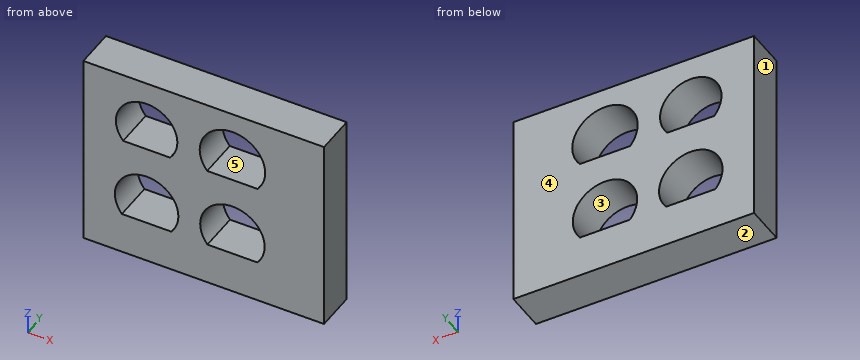
from build123d import *

# Parameters (mm, degrees)
SKETCH1_W           = 12.136372274
SKETCH1_H           = 9.961646607
BOSS_EXTRUDE2_DEPTH = 2


with BuildPart() as part:
    # Sketch1 → Boss-Extrude2 (new body)
    with BuildSketch(Plane(origin=(0, 0, 0), x_dir=(1, 0, 0), z_dir=(0, 1, 0))):
        with Locations((2.877549337, 2.284027555)):
            Rectangle(SKETCH1_W, SKETCH1_H)
        with BuildLine():
            Line((-1.184271928, 1), (1.184271928, 1))
            ThreePointArc((1.184271928, 1), (0, -1.55), (-1.184271928, 1))
        make_face(mode=Mode.SUBTRACT)
        with BuildLine():
            Line((3.05341377, 1), (5.598998182, 1))
            ThreePointArc((5.598998182, 1), (4.326205976, -1.7), (3.05341377, 1))
        make_face(mode=Mode.SUBTRACT)
        with BuildLine():
            Line((-1.2489996, 5.143134086), (1.2489996, 5.143134086))
            ThreePointArc((1.2489996, 5.143134086), (0, 2.543134086), (-1.2489996, 5.143134086))
        make_face(mode=Mode.SUBTRACT)
        with BuildLine():
            Line((3.065253955, 5.143134086), (5.587157997, 5.143134086))
            ThreePointArc((5.587157997, 5.143134086), (4.326205976, 2.493134086), (3.065253955, 5.143134086))
        make_face(mode=Mode.SUBTRACT)
    extrude(amount=BOSS_EXTRUDE2_DEPTH)


solid = part.part
Could you check a few things on this model? Use its own coordinates, in mm. Face numbers are marked on the shaded views. A direction names the side the tool comes from. Give positions to 0.01 mm unless a question says otherwise; leave off trailing zeros. Loops run counter-clockwise (first coordinate to the right, second up) from the corner with the lowest first, then second, coordinate; pieces in that order, holes last. Notation, with made-up numbers: M 7.5,-3 L 40.5,-3 A25 ccw 40.5,9 Z; hole C -24,43 d11. An arc over 180 degrees is marked long. Answer as a JSON object with one key per item and string values.
Q1. For the marked faces 4 and 5, which set-ups out of +Z, -Z, +X, -X, +Y, -Y let a thin tool reach every point of the face, with its end or its side?
Values found:
{"face 4": "+Z, -Z, +X, -X, +Y", "face 5": "+Y, -Y"}
Q2. Suppose I cut it at B-B, the plane y = 0.5. List the corners of the cut face in (x, z) for me (3 decimals).
Values found:
{"outline": "M -3.191,-7.265 L 8.946,-7.265 L 8.946,2.697 L -3.191,2.697 Z; hole M -1.249,-5.143 L 1.249,-5.143 A1.6 ccw long Z; hole M -1.184,-1 L 1.184,-1 A1.55 ccw long Z; hole M 3.053,-1 L 5.599,-1 A1.65 ccw long Z; hole M 3.065,-5.143 L 5.587,-5.143 A1.625 ccw long Z"}
Q3. If I drill on probe 1 along Z at (x, y) = (4.25, 1.75); probe 2 along X at (y, z) = (0.95, 0.05); probe 3 along X at (y, z) = (0.2, -5), over which ranges is the centre line in solid material (lowest first)? Write a range as [from, to].
Values found:
{"probe 1": "z = [-7.26, -5.14], [-2.49, -1], [1.7, 2.7]", "probe 2": "x = [-3.19, -1.55], [1.55, 2.68], [5.98, 8.95]", "probe 3": "x = [-3.19, -1.35], [1.35, 2.96], [5.69, 8.95]"}
Q4. Suppose I cut it at C-C, the plane z = 0.05. List the corners of the cut face in (x, y) for me, plus the area to 3 significant figures.
Values found:
{"outline": "M -3.19,0 L -1.55,0 L -1.55,2 L -3.19,2 Z; M 1.55,0 L 2.68,0 L 2.68,2 L 1.55,2 Z; M 5.98,0 L 8.95,0 L 8.95,2 L 5.98,2 Z", "area": "11.5 mm²"}
Q5. Suppose I cut it at A-A, the plane x = 0. List the corners of the cut face in (y, z) for me.
Values found:
{"outline": "M 0,-7.26 L 2,-7.26 L 2,-5.14 L 0,-5.14 Z; M 0,-2.54 L 2,-2.54 L 2,-1 L 0,-1 Z; M 0,1.55 L 2,1.55 L 2,2.7 L 0,2.7 Z"}
Q6. For P1, Ø4, axis at x = 4.33, z = 0.05, coming from the -Y side, with a flat end and sliding along its axis, tell me the tip position at first contact or that it passes through.
Values found:
{"P1": "stops at y = 0"}
Q7. If we mould it in two halves opening along X, with no side actions, what happens to the marked faces 1, 2 and 3? For each: pulls with the +X half, pulls with the -X half, needs draft (parallel to the pull), parting line crosses it, or undercut.
Values found:
{"face 1": "pulls with the -X half", "face 2": "needs draft", "face 3": "undercut"}
